from build123d import *

# Parameters (mm, degrees)
RESSALTO_EXTRUS_O1_DEPTH = 42
SKETCH5_W                = 30
SKETCH5_H                = 5
BOSS_EXTRUDE3_DEPTH      = 21
FILLET1_R                = 2.5
CHAMFER1_SIZE            = 1
ESBO_O2_R                = 1
CORTE_EXTRUS_O1_DEPTH    = 141.585462716


with BuildPart() as part:
    # Esboço1 → Ressalto-extrusão1 (new body)
    with BuildSketch(Plane.XY):
        with BuildLine():
            ThreePointArc((59.825652908, 72.25788881), (-0.070426749, 62.989274947), (-59.955692994, 72.327500038))
            Line((-59.955692994, 72.327500038), (-59.955692994, 69.181335803))
            ThreePointArc((-59.955692994, 69.181335803), (-51.505359903, 66.732393535), (-42.955692994, 64.656666352))
            Line((-42.955692994, 64.656666352), (-42.955692994, 60.00350113))
            Line((-42.955692994, 60.00350113), (43.044307006, 60.00350113))
            Line((43.044307006, 60.00350113), (43.044307006, 64.656666352))
            ThreePointArc((43.044307006, 64.656666352), (51.483258227, 66.702959658), (59.825652908, 69.112869408))
            Line((59.825652908, 69.112869408), (59.825652908, 72.25788881))
        make_face()
    extrude(amount=RESSALTO_EXTRUS_O1_DEPTH)

    # Sketch5 → Boss-Extrude3 (add)
    with BuildSketch(Plane.XY.offset(42)):
        with Locations((-27.955692994, 62.50350113)):
            Rectangle(SKETCH5_W, SKETCH5_H)
        with Locations((28.044307006, 62.50350113)):
            Rectangle(SKETCH5_W, SKETCH5_H)
    extrude(amount=BOSS_EXTRUDE3_DEPTH)

    # Fillet1
    fillet1_edges = [part.edges().sort_by_distance(p)[0] for p in [
        (-27.955692994, 65.00350113, 63),
        (-27.955692994, 60.00350113, 63),
        (28.044307006, 65.00350113, 63),
        (28.044307006, 60.00350113, 63),
    ]]
    fillet(fillet1_edges, radius=FILLET1_R - 0.0001)  # a hair under: the kernel refuses the full size

    # Chamfer1
    chamfer1_edges = [part.edges().sort_by_distance(p)[0] for p in [
        (0.044307006, 60.00350113, 42),
    ]]
    chamfer(chamfer1_edges, length=CHAMFER1_SIZE)

    # Esboço2 → Corte-extrusão1 (cut, through all)
    with BuildSketch(Plane.ZY.offset(42.955692994)):
        with Locations((60.5, 62.50350113)):
            Circle(ESBO_O2_R)
    extrude(amount=-CORTE_EXTRUS_O1_DEPTH, mode=Mode.SUBTRACT)


solid = part.part
Source: CAD feature listing. Evaluate the final solid. Frame: model axes, mm. A direction names the side the tool comes from. Round coordinates to 2 decimals unless told otherwise and drop trailing zeros. Order: outer loops, then holes, each group sorted by start corner. A loop starts at its lowest first (then second) coordinate and runs counter-clockwise, first axis right, second up. Notation, with made-up numbers: (-5, 60.5) - (14, 60.5) arc R25 ccw to (14, 89.5) - close; hole circle Ø9 at (58, -26). An arc over 180 degrees is marked (long way). Use a Markdown table: item, result. Add a question column.
1. First-contact query: pin 1 (0.5 mm diameter, centred on x = 19, y = 64.5, fed in from -Z); pin 2 (20.5 mm diameter, centred on x = 33, z = 55.5, fed in from +Y); pin 3 (4 mm diameter, centred on x = -25.5, z = 8.5, fed in from +Y); pin 4 (1.3 mm diameter, centred on x = -19, y = 64, fed in from -Z). Flat tips, straight axial feed; report the tip coordinate or a pass-through.
2. Section query D-D (x = -2). Return the cut outline in (y, z).
3. Section query C-C (z = 30). Return the cut outline in (x, y).
4. Line query: probe 1 along X at (y, z) = (64.5, 55); probe 2 along Y at (x, z) = (-30, 60.5); probe 3 along Z at (x, y) = (21, 62.5). Output: solid intervals per line, ascending.
5. Mould query, pull axis X, two halves, no side actions, for faces 1 (the cylindrical face through (-27.75, 60.72, 62.25)), 2 (the flat face through (13.044, 62, 52)), 3 (the flat face through (59.826, 71, 21)), 4 (the cylindrical face through (0.78, 62.99, 20.71)). Classes: +X half, -X half, draft (parallel to the pull), parting line (faces both ways), or undercut.
6. Set-up query: faces 5 (the flat face through (28, 65.004, 51)), 6 (the flat face through (-59.956, 71, 21)), 7 (the flat face through (0, 62, 42)). Return all of +Z, -Z, +X, -X, +Y, -Y with unobstructed straight access to the full face (end or side cutting, diameter ignored); none if empty.
7. Section query A-A (z = 47). Return the cut outline in (x, y).
Derived:
| question | item | result |
|---|---|---|
| 1 | pin 1 | z = 42 |
| 1 | pin 2 | y = 65 |
| 1 | pin 3 | y = 64.92 |
| 1 | pin 4 | z = 0 |
| 2 | outline | (60, 0) - (63, 0) - (63, 42) - (61, 42) - (60, 41) - close |
| 3 | outline | (-59.96, 69.18) arc R200.42 ccw to (-42.96, 64.66) - (-42.96, 60) - (43.04, 60) - (43.04, 64.66) arc R200.42 ccw to (59.83, 69.11) - (59.83, 72.26) arc R197.42 cw to (-59.96, 72.33) - close |
| 4 | probe 1 | -42.96 to -12.96, 13.04 to 43.04 |
| 4 | probe 2 | 60 to 61.5, 63.5 to 65 |
| 4 | probe 3 | 0 to 59.5, 61.5 to 63 |
| 5 | face 1 | draft |
| 5 | face 2 | undercut |
| 5 | face 3 | +X half |
| 5 | face 4 | undercut |
| 6 | face 5 | +Z, +X, -X, +Y |
| 6 | face 6 | +Z, -Z, -X, +Y, -Y |
| 6 | face 7 | +Z, +Y, -Y |
| 7 | outline | (-42.96, 60) - (-12.96, 60) - (-12.96, 65) - (-42.96, 65) - close; (13.04, 60) - (43.04, 60) - (43.04, 65) - (13.04, 65) - close |
